Read the model definition and answer for the solid it produces. Units are mm, in the model's axes. Give positions to 0.01 mm unless a question says otherwise; leave off trailing zeros. Order: outer loops, then holes, each group sorted by start corner. A loop starts at its lowest first (then second) coordinate and runs counter-clockwise, first axis right, second up.
Item 1: Find the intervals of material crossed by line 1 along Y through (x, z) = (47, 2.5); line 2 along X through (y, z) = (107.5, 6.25); line 3 along X through (y, z) = (146.05, 5), in increasing order.
Item 2: A cutting plane is placed at C-C (y = 63). Write down the section's boundary in (x, z), plus the area to 3 significant figures.
Item 3: Given pin 1 Ø3 at (x, z) = (207.5, 4) entering from +Y; pin 2 Ø3 at (x, z) = (173.5, 3) entering from -Y; pin 3 Ø1.9 at (x, z) = (3, 3) entering from -Y (3 decimals), each flat-ended and moving along its own axis, determine where each tip first touches the part or whether it passes through.
Item 4: A cutting plane is placed at B-B (x = 202). Write down the section's boundary in (y, z), plus the area to 3 significant figures.
Item 5: A cutting plane is placed at A-A (y = 146.05). Write down the section's boundary in (x, z).
Item 6: A cutting plane is placed at D-D (z = 1.25). State how many separate pieces and enclosed holes the cut face has, plus the area to 3 significant figures.
from build123d import *

# Parameters (mm, degrees)
BOSS_EXTRUDE1_DEPTH          = 6.35
SKETCH2_W                    = 127
SKETCH2_H                    = 19.05
CUT_EXTRUDE1_DEPTH           = 195.543611155
SKETCH3_W                    = 86.864773719
SKETCH3_H                    = 114.3
BOSS_EXTRUDE2_DEPTH          = 6.35
SKETCH4_W                    = 6.35
SKETCH4_H                    = 9.525
SKETCH4_H_2                  = 44.45
SKETCH4_H_3                  = 15.875
CUT_EXTRUDE2_DEPTH           = 253.93516292
SKETCH5_W                    = 19.05
SKETCH5_H                    = 6.35
BOSS_EXTRUDE3_DEPTH          = 6.35
BOSS_EXTRUDE4_DEPTH          = 6.35
LPATTERN1_COUNT              = 2
LPATTERN1_PITCH              = 50.8
F_10_0_1935_DIAMETER_HOLE1_D = 4.9149
F_10_0_1935_DIAMETER_HOLE2_D = 4.9149
BOSS_EXTRUDE8_DEPTH          = 6.35
CUT_EXTRUDE4_DEPTH           = 283.81411342
FILLET1_R                    = 2.54


with BuildPart() as part:
    # Sketch1 → Boss-Extrude1 (new body)
    with BuildSketch(Plane.XY):
        Polygon((86.864773719, 57.15), (185.851477372, 0), (86.864773719, 0), (0, 0), (0, 57.15), align=None)
    extrude(amount=BOSS_EXTRUDE1_DEPTH)

    # Sketch2 → Cut-Extrude1 (cut, through all)
    with BuildSketch(Plane.XY.offset(6.35)):
        with Locations((69.85, 9.525)):
            Rectangle(SKETCH2_W, SKETCH2_H)
    extrude(amount=-CUT_EXTRUDE1_DEPTH, mode=Mode.SUBTRACT)

    # Sketch3 → Boss-Extrude2 (add)
    with BuildSketch(Plane.XY.offset(6.35)):
        with Locations((43.432386859, 114.3)):
            Rectangle(SKETCH3_W, SKETCH3_H)
    extrude(amount=-BOSS_EXTRUDE2_DEPTH)

    # Sketch4 → Cut-Extrude2 (cut, through all)
    with BuildSketch(Plane.XY.offset(6.35)):
        with Locations((3.175, 4.7625)):
            Rectangle(SKETCH4_W, SKETCH4_H)
        with Locations((3.175, 50.8)):
            Rectangle(SKETCH4_W, SKETCH4_H_2)
        with Locations((3.175, 114.3)):
            Rectangle(SKETCH4_W, SKETCH4_H_2)
        with Locations((3.175, 163.5125)):
            Rectangle(SKETCH4_W, SKETCH4_H_3)
    extrude(amount=-CUT_EXTRUDE2_DEPTH, mode=Mode.SUBTRACT)

    # Sketch5 → Boss-Extrude3 (add)
    with BuildSketch(Plane.XY.offset(6.35)):
        with Locations((158.75, -3.175)):
            Rectangle(SKETCH5_W, SKETCH5_H)
    extrude(amount=-BOSS_EXTRUDE3_DEPTH)

    # Sketch6 → Boss-Extrude4 (add)
    with BuildSketch(Plane.XY.offset(6.35)):
        Polygon((108.861818976, 44.45), (125.359602918, 34.925), (128.534602918, 40.424261314), (112.036818976, 49.949261314), align=None)
    boss_extrude4 = extrude(amount=-BOSS_EXTRUDE4_DEPTH)

    # LPattern1: Boss-Extrude4 ×2
    with Locations(*[Vector(0.8660254037844415, -0.49999999999999517, 0) * (i * LPATTERN1_PITCH) for i in range(1, LPATTERN1_COUNT)]):
        add(boss_extrude4)

    # #10 (0.1935) Diameter Hole1 (through all)
    with Locations(Plane.XY.offset(6.35)):
        with Locations((3.175, 146.05), (3.175, 82.55), (3.175, 19.05)):
            Hole(F_10_0_1935_DIAMETER_HOLE1_D / 2)

    # #10 (0.1935) Diameter Hole2 (through all)
    with Locations(Plane.XY.offset(6.35)):
        with Locations((118.698210947, 42.437130657), (162.692301459, 17.037130657), (158.75, -3.175)):
            Hole(F_10_0_1935_DIAMETER_HOLE2_D / 2)

    # Sketch20 → Boss-Extrude8 (add)
    with BuildSketch(Plane.XY.offset(6.35)):
        Polygon((172.52869343, 15.024261314), (189.026477372, 5.499261314), (214.426477372, 5.499261314), (224.829708334, 12.783682056), (224.829708334, 0.934420742), (214.426477372, -6.35), (185.851477372, -6.35), (184.15, -6.35), (184.15, 0), (185.851477372, 0), (169.35369343, 9.525), align=None)
    extrude(amount=-BOSS_EXTRUDE8_DEPTH)

    # Sketch22 → Cut-Extrude4 (cut, through all)
    with BuildSketch(Plane.XY.offset(6.35)):
        Polygon((17.220652064, 161.925), (17.220652064, 79.375), (43.43238686, 120.65), align=None)
        Polygon((75.994121656, 79.375), (49.78238686, 120.65), (75.994121656, 161.925), align=None)
        Polygon((21.20738686, 164.45678038), (46.60738686, 124.46), (72.00738686, 164.45678038), align=None)
        Polygon((46.60738686, 116.84), (72.00738686, 76.84321962), (21.20738686, 76.84321962), align=None)
    extrude(amount=-CUT_EXTRUDE4_DEPTH, mode=Mode.SUBTRACT)

    # Fillet1
    fillet1_edges = [part.edges().sort_by_distance(p)[0] for p in [
        (17.220652064, 161.925, 3.175),
        (43.43238686, 120.65, 3.175),
        (17.220652064, 79.375, 3.175),
        (75.994121656, 161.925, 3.175),
        (75.994121656, 79.375, 3.175),
        (49.78238686, 120.65, 3.175),
        (21.20738686, 164.45678038, 3.175),
        (72.00738686, 164.45678038, 3.175),
        (46.60738686, 124.46, 3.175),
        (21.20738686, 76.84321962, 3.175),
        (46.60738686, 116.84, 3.175),
        (72.00738686, 76.84321962, 3.175),
    ]]
    fillet(fillet1_edges, radius=FILLET1_R)


solid = part.part
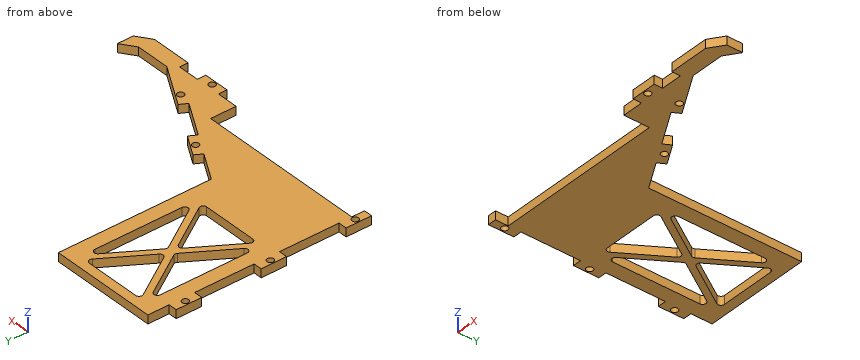
Response values:
1. line 1: y = 19.05 to 76.84, 114.61 to 126.69, 164.46 to 171.45
1. line 2: x = 6.35 to 17.22, 35.08 to 40.68, 52.54 to 58.13, 75.99 to 86.86
1. line 3: x = 0 to 0.72, 5.63 to 17.22, 27.3 to 32.9, 60.32 to 65.91, 75.99 to 86.86
2. outline: (6.35, 0) - (86.86, 0) - (86.86, 6.35) - (6.35, 6.35) - close
2. area: 511 mm2
3. pin 1: stops at y = 5.5
3. pin 2: stops at y = 0
3. pin 3: stops at y = 9.525
4. outline: (-6.35, 0) - (5.5, 0) - (5.5, 6.35) - (-6.35, 6.35) - close
4. area: 75.2 mm2
5. outline: (0, 0) - (0.72, 0) - (0.72, 6.35) - (0, 6.35) - close; (5.63, 0) - (17.22, 0) - (17.22, 6.35) - (5.63, 6.35) - close; (27.3, 0) - (32.9, 0) - (32.9, 6.35) - (27.3, 6.35) - close; (60.32, 0) - (65.91, 0) - (65.91, 6.35) - (60.32, 6.35) - close; (75.99, 0) - (86.86, 0) - (86.86, 6.35) - (75.99, 6.35) - close
6. separate pieces: 1
6. enclosed holes: 10
6. area: 11,300 mm2
